```python
from build123d import *

# Parameters (mm, degrees)
SKETCH1_W           = 6
SKETCH1_H           = 6
BOSS_EXTRUDE1_DEPTH = 4
SKETCH2_R           = 1.75
BOSS_EXTRUDE2_DEPTH = 1.25
SKETCH3_W           = 1.5
SKETCH3_H           = 1
BOSS_EXTRUDE3_DEPTH = 5


with BuildPart() as part:
    # Sketch1 → Boss-Extrude1 (new body)
    with BuildSketch(Plane(origin=(0, 0, 0), x_dir=(1, 0, 0), z_dir=(0, 1, 0))):
        Rectangle(SKETCH1_W, SKETCH1_H)
    extrude(amount=BOSS_EXTRUDE1_DEPTH)

    # Sketch2 → Boss-Extrude2 (add)
    with BuildSketch(Plane(origin=(0, 4, 0), x_dir=(1, 0, 0), z_dir=(0, 1, 0))):
        with Locations(Location((0, 0, 0), (0, 0, 270))):
            Circle(SKETCH2_R)
    extrude(amount=BOSS_EXTRUDE2_DEPTH)

    # Sketch3 → Boss-Extrude3 (add)
    with BuildSketch(Plane.XZ):
        with Locations((2.25, 0)):
            Rectangle(SKETCH3_W, SKETCH3_H)
        with Locations((-2.25, 0)):
            Rectangle(SKETCH3_W, SKETCH3_H)
    extrude(amount=BOSS_EXTRUDE3_DEPTH)


solid = part.part
```
Input: part model. Units: mm. Frame: model coordinates. A direction names the side the tool comes from. Coordinates: 2 decimals unless noted, no trailing zeros. Write each loop counter-clockwise with the first axis right and the second up, starting at its lowest first coordinate (ties: lowest second). Pieces come first, ordered by that corner, then holes. Notation, with made-up numbers: (89, -30.75) - (143, -30.75) arc R35 ccw to (143, 1.25) - close; hole circle Ø10 at (74.5, 88.5). An arc over 180 degrees is marked (long way). Put each result on its own line as item: value. Start each with the question number.
1) Cut plane C-C (z = 0). Return the cut outline in (x, y).
2) Mould query, pull axis X, two halves, no side actions, for faces 5 (the face through (-1.5, -2, 0)), 6 (the face through (1.5, -2, 0)), 7 (the face through (3, 1, 0)), 8 (the face through (-2, -2, 0.5)). Classes: pulls with the +X half, pulls with the -X half, needs draft (parallel to the pull), parting line crosses it, or undercut.
3) Cut plane A-A (y = -0.75). Return the cut outline in (x, z), plus the area to 3 significant figures.
4) Reachability of faces 1 (the face through (-2, -2, -0.5)), 2 (the face through (1.3, 4, -1.4)), 3 (the face through (2, -2, 0.5)), 4 (the face through (-2, -5, 0)) from +Z, -Z, +X, -X, +Y, -Y: full face, straight path, thin tool, end or side. Return the list, or none.
5) Ray query, L1, parallel to X at y = -2.5, z = 0.35; L2, parallel to Y at x = -0.35, z = 1.45; L3, parallel to Y at x = 1.65, z = -2.6. Return the intervals inside material, ascending.
6) Contact query for flat-ended pins moving along their axis: pin 1 (2 mm diameter, centred on x = 1.5, z = 2, fed in from -Y); pin 2 (3 mm diameter, centred on x = 2, y = -2.5, fed in from -Z); pin 3 (0.8 mm diameter, centred on x = -2.5, y = -3.5, fed in from +Z). Output: stop coordinate, or through.
7) Cut plane B-B (x = 2.5). Return the cut outline in (y, z).
8) Cut plane D-D (x = 0). Return the cut outline in (y, z), plus the area to 3 significant figures.
Resolved:
1. outline: (-3, -5) - (-1.5, -5) - (-1.5, 0) - (1.5, 0) - (1.5, -5) - (3, -5) - (3, 4) - (1.75, 4) - (1.75, 5.25) - (-1.75, 5.25) - (-1.75, 4) - (-3, 4) - close
2. face 5: undercut
2. face 6: undercut
2. face 7: pulls with the +X half
2. face 8: needs draft
3. outline: (-3, -0.5) - (-1.5, -0.5) - (-1.5, 0.5) - (-3, 0.5) - close; (1.5, -0.5) - (3, -0.5) - (3, 0.5) - (1.5, 0.5) - close
3. area: 3.00 mm2
4. face 1: -Z, +X, -X, -Y
4. face 2: +Y
4. face 3: +Z, +X, -X, -Y
4. face 4: +Z, -Z, +X, -X, -Y
5. L1: x = -3 to -1.5, 1.5 to 3
5. L2: y = 0 to 5.25
5. L3: y = 0 to 4
6. pin 1: stops at y = 0
6. pin 2: stops at z = -0.5
6. pin 3: stops at z = 0.5
7. outline: (-5, -0.5) - (0, -0.5) - (0, -3) - (4, -3) - (4, 3) - (0, 3) - (0, 0.5) - (-5, 0.5) - close
8. outline: (0, -3) - (4, -3) - (4, -1.75) - (5.25, -1.75) - (5.25, 1.75) - (4, 1.75) - (4, 3) - (0, 3) - close
8. area: 28.4 mm2
